```python
from build123d import *

# Parameters (mm, degrees)
F0_W     = 50
F0_H     = 30
F1_DEPTH = 30
F3_DEPTH = 50
F5_DEPTH = 30
F7_DEPTH = 15
F6_W     = 20
F6_H     = 10
F8_DEPTH = 20
F9_SIZE  = 10


with BuildPart() as f1:
    # F0 (on Front) → F1 (new body)
    with BuildSketch(Plane.XZ):
        with Locations((-25, 15)):
            Rectangle(F0_W, F0_H)
    extrude(amount=F1_DEPTH)

    # F2 (on face) → F3 (cut, through all)
    with BuildSketch(Plane.YZ):
        with BuildLine():
            Line((-30, 0), (-22.5, 0))
            ThreePointArc((-22.5, 0), (-24.6966991411, 5.3033008589), (-30, 7.5))
            Line((-30, 7.5), (-30, 0))
        make_face()
    extrude(amount=-F3_DEPTH, mode=Mode.SUBTRACT)

    # F4 (on face) → F5 (cut, through all)
    with BuildSketch(Plane.XY.offset(30)):
        with BuildLine():
            Line((0, 0), (-10, 0))
            ThreePointArc((-10, 0), (-7.0710678119, -7.0710678119), (0, -10))
            Line((0, -10), (0, 0))
        make_face()
    extrude(amount=-F5_DEPTH, mode=Mode.SUBTRACT)

    # F6 (on face) → F7 (cut)
    with BuildSketch(Plane.XZ.offset(30)):
        with BuildLine():
            Line((0, 30), (-7.5, 30))
            ThreePointArc((-7.5, 30), (-5.3033008589, 24.6966991411), (0, 22.5))
            Line((0, 22.5), (0, 30))
        make_face()
    extrude(amount=-F7_DEPTH, mode=Mode.SUBTRACT)

    # F6 (on face) → F8 (cut)
    with BuildSketch(Plane.XZ.offset(30)):
        with Locations((-25, 15)):
            Rectangle(F6_W, F6_H)
    extrude(amount=-F8_DEPTH, mode=Mode.SUBTRACT)

    # F9
    f9_edges = [f1.edges().sort_by_distance(p)[0] for p in [
        (-50, -15, 30),
    ]]
    chamfer(f9_edges, length=F9_SIZE)


solid = f1.part
```
Input: part model. Units: mm. Frame: model coordinates. A direction names the side the tool comes from. Give positions to 0.01 mm unless a question says otherwise; leave off trailing zeros. Order: outer loops, then holes, each group sorted by start corner. A loop starts at its lowest first (then second) coordinate and runs counter-clockwise, first axis right, second up. Notation, with made-up numbers: (26, 85) - (35, 85) arc R20 cw to (35, 116) - close; hole circle Ø10 at (28, -27.75). An arc over 180 degrees is marked (long way). Put each result on its own line as item: value.
Item 1: Draft query along X for faces 1 (the flat face through (-45, -15, 25)), 2 (the flat face through (-15, -20, 15)), 3 (the flat face through (-35, -20, 15)), 4 (the cylindrical face through (-24.65, -24.639, 5.245)). Return one class per face: +X half, -X half, draft (parallel to the pull), parting line (faces both ways), or undercut.
Found:
face 1: -X half
face 2: undercut
face 3: undercut
face 4: draft
Item 2: Section query B-B, the plane x = -17.5. Return loops of the section in (y, z), then the cut area to 3 significant figures.
Found:
outline: (-30, 7.5) arc R7.5 cw to (-22.5, 0) - (0, 0) - (0, 30) - (-30, 30) - (-30, 20) - (-10, 20) - (-10, 10) - (-30, 10) - close
area: 656 mm^2
Item 3: Section query A-A, the plane y = -19. Return loops of the section in (x, z), then the cut area to 3 significant figures.
Found:
outline: (-50, 0) - (0, 0) - (0, 22.5) arc R7.5 cw to (-7.5, 30) - (-40, 30) - (-50, 20) - close; hole (-35, 10) - (-15, 10) - (-15, 20) - (-35, 20) - close
area: 1,210 mm^2
Item 4: Contact query for flat-ended pins moving along their axis: pin 1 (6 mm diameter, centred on y = -13, z = 25, fed in from -X); pin 2 (5 mm diameter, centred on x = -27, z = 15.5, fed in from -Y). Output: stop coordinate, or through.
Found:
pin 1: stops at x = -48
pin 2: stops at y = -10
Item 5: Section query C-C, the plane z = 16.25. Return loops of the section in (x, y), then the cut area to 3 significant figures.
Found:
outline: (-50, -30) - (-35, -30) - (-35, -10) - (-15, -10) - (-15, -30) - (0, -30) - (0, -10) arc R10 cw to (-10, 0) - (-50, 0) - close
area: 1,020 mm^2
Item 6: Access query for faces 5 (the flat face through (-30, 0, 15)), 6 (the flat face through (-3, -15, 27)), 7 (the flat face through (-25, -20, 20)). Directions: +Z, -Z, +X, -X, +Y, -Y. A direction counts if a zero-diameter tool reaches every point of the face in a straight line with its end or side. Return the directions, or none.
Found:
face 5: +Z, -Z, +X, -X, +Y
face 6: +Z, +X, -Y
face 7: -Y
Item 7: Section query D-D, the plane y = -11.5. Return loops of the section in (x, z).
Found:
outline: (-50, 0) - (0, 0) - (0, 30) - (-40, 30) - (-50, 20) - close; hole (-35, 10) - (-15, 10) - (-15, 20) - (-35, 20) - close
Item 8: Ray query, L1, parallel to X at y = -23.5, z = 18; L2, parallel to Y at x = -16.5, z = 16.25; L3, parallel to Z at x = -17, y = -17.25. Return the intervals inside material, ascending. Write a range as from..to.
Found:
L1: x = -50..-35, -15..0
L2: y = -10..0
L3: z = 0..10, 20..30
